Check sheet for the modelled part. Datum: model origin and axes. Units: mm. A direction names the side the tool comes from. Give positions to 0.01 mm unless a question says otherwise; leave off trailing zeros. Loops run counter-clockwise (first coordinate to the right, second up) from the corner with the lowest first, then second, coordinate; pieces in that order, holes last. Notation, with made-up numbers: (-16.5, 41.25) - (33.5, 41.25) arc R24 ccw to (33.5, 75.25) - close; hole circle Ø6 at (47.5, -7.5). An arc over 180 degrees is marked (long way). Answer in a Markdown table with one row per item. Add a question column.
(1) Set-up check for faces 4 (the face through (1, -15, 20)), 5 (the face through (49, -30, -37)), 6 (the face through (100, -60, -1)): record each of +Z, -Z, +X, -X, +Y, -Y from which the full face is reachable in a straight line by a thin tool's end or side.
(2) Go/stop test with flat-tipped pins: P1, Ø1, axis at x = 55, z = 14, coming from the -Y side; P2, Ø1.5, axis at x = 42, z = -7.5, coming from the +Y side; P3, Ø1, axis at x = 59, z = 32, coming from the +Y side. Record where each tip stops, or that it passes through.
(3) Draft check along X on faces 1 (the face through (98, -50, 0)), 2 (the face through (0, -60, -1)), 3 (the face through (3, -59, -1)). Enter one of: released by +X, released by -X, zero draft, split by the parting line, or undercut.
(4) Sectioned sample at D-D on y = -36.5. Enter the section's corners in (x, z).
(5) Sectioned sample at A-A on x = 6. Enter the section's corners in (y, z).
(6) Sectioned sample at C-C on z = -1. Enter the section's corners in (x, y).
(7) Thickness scan on L1, parallel to Z at x = 21.5, y = -13.5; L2, parallel to X at y = -50.5, z = 27.5; L3, parallel to Y at x = 47.5, z = 1. Record the ranges inside material, lowest first.
(8) Sectioned sample at B-B on y = -53.5. Enter the section's corners in (x, z).
from build123d import *

# Parameters (mm, degrees)
BOSS_EXTRUDE2_DEPTH = 100
SHELL1_T            = -3


with BuildPart() as part:
    # Sketch1 → Boss-Extrude2 (new body)
    with BuildSketch(Plane(origin=(0, 0, 0), x_dir=(0, 0, -1), z_dir=(1, 0, 0))):
        with BuildLine():
            Line((40, 0), (40, -60))
            ThreePointArc((40, -60), (0, -100), (-40, -60))
            Line((-40, -60), (-40, 0))
            Line((-40, 0), (-20, 0))
            Line((-20, 0), (-20, -30))
            ThreePointArc((-20, -30), (0, -50), (20, -30))
            Line((20, -30), (20, 0))
            Line((20, 0), (40, 0))
        make_face()
    extrude(amount=BOSS_EXTRUDE2_DEPTH)

    # Shell1
    shell1_openings = [part.faces().sort_by_distance(p)[0] for p in [
        (50, 0, -30),
        (50, -15, -20),
        (50, -50, 0),
        (50, -15, 20),
        (50, 0, 30),
    ]]
    offset(amount=SHELL1_T, openings=shell1_openings, kind=Kind.INTERSECTION)


solid = part.part
Reply:
| question | item | result |
|---|---|---|
| 1 | face 4 | +X, -X, +Y |
| 1 | face 5 | +Y |
| 1 | face 6 | +Z, -Z, +X, +Y, -Y |
| 2 | P1 | y = -97.65 |
| 2 | P2 | y = -96.07 |
| 2 | P3 | y = -77.68 |
| 3 | face 1 | zero draft |
| 3 | face 2 | released by -X |
| 3 | face 3 | undercut |
| 4 | outline | (0, -40) - (100, -40) - (100, -18.91) - (97, -18.91) - (97, -37) - (3, -37) - (3, -18.91) - (0, -18.91) - close; (0, 18.91) - (3, 18.91) - (3, 37) - (97, 37) - (97, 18.91) - (100, 18.91) - (100, 40) - (0, 40) - close |
| 5 | outline | (-60, -40) - (0, -40) - (0, -37) - (-60, -37) arc R37 cw to (-60, 37) - (0, 37) - (0, 40) - (-60, 40) arc R40 ccw to start |
| 6 | outline | (0, -99.99) - (100, -99.99) - (100, -49.97) - (97, -49.97) - (97, -96.99) - (3, -96.99) - (3, -49.97) - (0, -49.97) - close |
| 7 | L1 | -40 to -37, 37 to 40 |
| 7 | L2 | 0 to 3, 97 to 100 |
| 7 | L3 | -99.99 to -96.99 |
| 8 | outline | (0, -40) - (100, -40) - (100, 40) - (0, 40) - close; hole (3, -37) - (97, -37) - (97, 37) - (3, 37) - close |
